Work out the finished part from the listing and answer in its coordinate system (mm). Coordinates: 2 decimals unless noted, no trailing zeros. Order: outer loops, then holes, each group sorted by start corner. A loop starts at its lowest first (then second) coordinate and runs counter-clockwise, first axis right, second up. Notation, with made-up numbers: M 0,54.25 L 14,54.25 A23 cw 14,65.25 Z; hole C 21.5,60 d2. An arc over 180 degrees is marked long. Use a Markdown table: item, result.
from build123d import *

# Parameters (mm, degrees)
SKETCH1_R           = 6.05
BOSS_EXTRUDE1_DEPTH = 7
SKETCH3_R           = 1.7
CUT_EXTRUDE2_DEPTH  = 60


with BuildPart() as part:
    # Sketch1 → Boss-Extrude1 (new body)
    with BuildSketch(Plane(origin=(0, 0, 0), x_dir=(1, 0, 0), z_dir=(0, 1, 0))):
        with BuildLine():
            Line((-86.41, -26.165178012), (-86.41, -43.765178012))
            Line((-86.41, -43.765178012), (-53.34, -43.765178012))
            Line((-53.34, -43.765178012), (-53.34, -26.165178012))
            Line((-53.34, -26.165178012), (-45.34, -26.165178012))
            Line((-45.34, -26.165178012), (-45.34, -48.765178012))
            Line((-45.34, -48.765178012), (-62.375, -48.765178012))
            Line((-62.375, -48.765178012), (-62.375, -97.765178012))
            Line((-62.375, -97.765178012), (37.625, -97.765178012))
            Line((37.625, -97.765178012), (71.6, -63.790178012))
            Line((71.6, -63.790178012), (86.215, -64.175178012))
            Line((86.215, -64.175178012), (86.215, -112.765178012))
            Line((86.215, -112.765178012), (66.349963518, -112.765178012))
            Line((66.349963518, -112.765178012), (73.821063238, -106.783510987))
            ThreePointArc((73.821063238, -106.783510987), (79.369481987, -101.331578198), (72.140531111, -104.203997211))
            Line((72.140531111, -104.203997211), (61.447619718, -112.765178012))
            Line((61.447619718, -112.765178012), (37.625, -112.765178012))
            Line((37.625, -112.765178012), (-77.375, -112.765178012))
            Line((-77.375, -112.765178012), (-77.375, -48.765178012))
            Line((-77.375, -48.765178012), (-94.41, -48.765178012))
            Line((-94.41, -48.765178012), (-94.41, -26.165178012))
            Line((-94.41, -26.165178012), (-86.41, -26.165178012))
        make_face()
        with Locations(Location((64.6, -90.765178012, 0), (0, 0, 270))):
            Circle(SKETCH1_R, mode=Mode.SUBTRACT)
    extrude(amount=BOSS_EXTRUDE1_DEPTH)

    # Sketch3 → Cut-Extrude2 (cut)
    with BuildSketch(Plane(origin=(-45.34, 0, 0), x_dir=(0, 0, -1), z_dir=(1, 0, 0))):
        with Locations((-31.065178012, 3.5)):
            Circle(SKETCH3_R)
    extrude(amount=-CUT_EXTRUDE2_DEPTH, mode=Mode.SUBTRACT)


solid = part.part
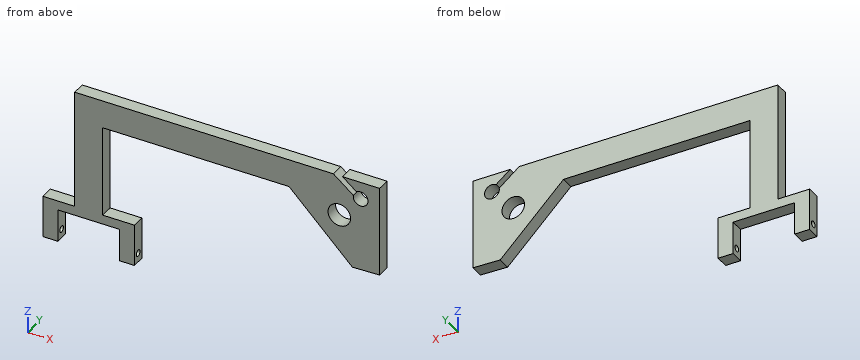
1. Section D-D on x = 64.6 is taken. Determine the outline of the cut face in (y, z).
Answers below:
| item | result |
|---|---|
| outline | M 0,70.79 L 7,70.79 L 7,84.72 L 0,84.72 Z; M 0,96.82 L 7,96.82 L 7,110.24 L 0,110.24 Z |
2. Section C-C on z = 39 is taken. Determine the outline of the cut face in (x, y), then the cut area to 3 significant figures.
Answers below:
| item | result |
|---|---|
| outline | M -94.41,0 L -86.41,0 L -86.41,7 L -94.41,7 Z; M -53.34,0 L -45.34,0 L -45.34,7 L -53.34,7 Z |
| area | 112 mm² |
3. Section A-A on y = 3.5 is taken. Give the number of separate pieces and of enclosed holes in the cut face, then the cut area to 3 significant figures.
Answers below:
| item | result |
|---|---|
| separate pieces | 3 |
| enclosed holes | 1 |
| area | 4,530 mm² |
4. Find the intervals of material crossed by probe 1 along Z at (x, y) = (-57.5, 6); probe 2 along X at (y, z) = (5.5, 98.5) (3 decimals); probe 3 along Z at (x, y) = (23, 3), in increasing order.
Answers below:
| item | result |
|---|---|
| probe 1 | 43.77 to 48.77, 97.77 to 112.77 |
| probe 2 | -77.375 to 86.215 |
| probe 3 | 97.77 to 112.77 |
5. Section B-B on z = 90 is taken. Determine the outline of the cut face in (x, y) (3 decimals).
Answers below:
| item | result |
|---|---|
| outline | M -77.375,0 L -62.375,0 L -62.375,7 L -77.375,7 Z; M 45.39,0 L 58.599,0 L 58.599,7 L 45.39,7 Z; M 70.601,0 L 86.215,0 L 86.215,7 L 70.601,7 Z |
6. Flat-ended cylindrical pins translate along their axes: P1, Ø3.5, axis at x = -63, y = 5, coming from the -Z side; P2, Ø1.5, axis at x = 67.5, y = 3.5, coming from the -Z side; P3, Ø4, axis at y = 3.5, z = 31.07, coming from the +X side. Find the tip coordinate at first contact, or state that the pin passes through.
Answers below:
| item | result |
|---|---|
| P1 | z = 43.77 |
| P2 | z = 67.14 |
| P3 | x = -45.34 |
